```python
from build123d import *

# Parameters (mm, degrees)
F0_W           = 203.2
F0_H           = 88.9
F1_DEPTH       = 2.54
F2_W           = 2.54
F2_H           = 26.416
F2_H_2         = 2.54
F2_W_2         = 16.764
F2_W_3         = 26.416
F3_DEPTH       = 20.32
F5_D           = 3.048
F5_CSINK_D     = 5.08
F5_CSINK_ANGLE = 49
F2_W_4         = 85.8261585236
F2_H_3         = 19.05
F6_DEPTH       = 25.4
F7_SIZE2       = 19.5063104746
F7_SIZE        = 15.24


with BuildPart() as f1:
    # F0 (on Top) → F1 (new body)
    with BuildSketch(Plane.XY):
        Rectangle(F0_W, F0_H)
    extrude(amount=F1_DEPTH)

    # F2 (on face) → F3 (join)
    with BuildSketch(Plane.XY.offset(2.54)):
        with Locations((-33.782, -31.242)):
            Rectangle(F2_W, F2_H)
        with Locations((-53.086, -31.242)):
            Rectangle(F2_W, F2_H)
        with Locations((-53.086, -16.764)):
            Rectangle(F2_W, F2_H_2)
        with Locations((33.782, -31.242)):
            Rectangle(F2_W, F2_H)
        with Locations((53.086, -31.242)):
            Rectangle(F2_W, F2_H)
        with Locations((53.086, -16.764)):
            Rectangle(F2_W, F2_H_2)
        with Locations((-24.13, -16.764)):
            Rectangle(F2_W_2, F2_H_2)
        with Locations((-14.478, -16.764)):
            Rectangle(F2_W, F2_H_2)
        with Locations((24.13, -16.764)):
            Rectangle(F2_W_2, F2_H_2)
        with Locations((14.478, -16.764)):
            Rectangle(F2_W, F2_H_2)
        with Locations((-33.782, -16.764)):
            Rectangle(F2_W, F2_H_2)
        with Locations((-43.434, -16.764)):
            Rectangle(F2_W_2, F2_H_2)
        with Locations((33.782, -16.764)):
            Rectangle(F2_W, F2_H_2)
        with Locations((43.434, -16.764)):
            Rectangle(F2_W_2, F2_H_2)
        with Locations((0, -16.764)):
            Rectangle(F2_W_3, F2_H_2)
        Polygon((13.208, -37.338), (13.208, -44.45), (15.748, -44.45), (15.748, -18.034), (13.208, -18.034), (13.208, -34.798), align=None)
        Polygon((-15.748, -18.034), (-15.748, -44.45), (-13.208, -44.45), (-13.208, -37.338), (-13.208, -34.798), (-13.208, -18.034), align=None)
        with Locations((0, -36.068)):
            Rectangle(F2_W_3, F2_H_2)
    extrude(amount=F3_DEPTH)

    # F5 (through all)
    with Locations(Plane(origin=(0, 0, 0), x_dir=(1, 0, 0), z_dir=(0, 0, -1))):
        with Locations((97.155, -40.005), (97.155, 40.005), (-97.155, 40.005), (-97.155, -40.005)):
            CounterSinkHole(F5_D / 2, F5_CSINK_D / 2, counter_sink_angle=F5_CSINK_ANGLE)

    # F2 (on face) → F6 (join)
    with BuildSketch(Plane.XY.offset(2.54)):
        with Locations((0, 34.925)):
            Rectangle(F2_W_4, F2_H_3)
    extrude(amount=F6_DEPTH)

    # F7
    f7_edges = [f1.edges().sort_by_distance(p)[0] for p in [
        (0, 25.4, 27.94),
    ]]
    f7_side = f1.faces().sort_by_distance((0, 34.925, 27.94))[0]
    chamfer(f7_edges, length=F7_SIZE, length2=F7_SIZE2, reference=f7_side)


solid = f1.part
```
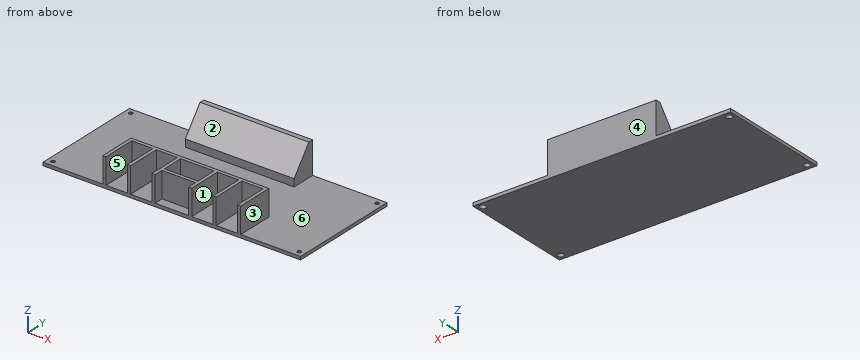
Design review of the part built by this model. Coordinates are the model's own, in mm. Face numbers are marked on the shaded views. A direction names the side the tool comes from. Round coordinates to 2 decimals unless told otherwise and drop trailing zeros. Write each loop counter-clockwise with the first axis right and the second up, starting at its lowest first coordinate (ties: lowest second). Pieces come first, ordered by that corner, then holes. Notation, with made-up numbers: (-35.5, -37.5) -> (-10.5, -37.5) arc R7 cw to (-10.5, -29.5) -> close; hole circle Ø4 at (-17, 40.5). An arc over 180 degrees is marked (long way). Write item = value, one per line. Start each with the question number.
1) Mouldability with a two-part tool opening along Y and no side actions: class the marked faces 4, 5 and 6 as +Y half, -Y half, draft (parallel to the pull), parting line (faces both ways), or undercut.
2) Take a section at C-C, the plane y = 29. State the section outline as (x, z) points, plus the area to 3 significant figures.
3) Clearance check with flat-ended pins moving along their axes: pin 1 (13.5 mm diameter, centred on x = -42, y = -31.5, fed in from +Z); pin 2 (2 mm diameter, centred on y = -22.5, z = 7, fed in from +X); pin 3 (6 mm diameter, centred on y = -32, z = 9, fed in from -X); pin 4 (13.5 mm diameter, centred on x = 26, z = 8.5, fed in from -Y). State where each tip first meets the part, or that it passes through.
4) Wall thickness on probe 1 along X at (y, z) = (-23, 7); probe 2 along X at (y, z) = (34, 9); probe 3 along Z at (x, y) = (75, -37): over which ranges is each line inside the solid? List them lowest first. Write a range as from..to.
5) Take a section at D-D, the plane y = -20. State the section outline as (x, z) points, plus the area to 3 significant figures.
6) Tool access review of the marked faces 1, 2 and 3: name each direction out of +Z, -Z, +X, -X, +Y, -Y from which nothing blocks a thin tool from reaching the whole face with its end or side.
7) Take a section at B-B, the plane x = 41. State the section outline as (y, z) points, plus the area to 3 significant figures.
8) Take a section at A-A, the plane z = 15.75. Count the separate pieces of the cut face and the enclosed holes in it, plus the area to 3 significant figures.
Results list:
q1.face_4 = +Y half
q1.face_5 = draft
q1.face_6 = undercut
q2.outline = (-101.6, 0) -> (101.6, 0) -> (101.6, 2.54) -> (42.91, 2.54) -> (42.91, 13.04) -> (-42.91, 13.04) -> (-42.91, 2.54) -> (-101.6, 2.54) -> close
q2.area = 1,420 mm²
q3.pin_1 = 2.54
q3.pin_2 = 54.36
q3.pin_3 = -54.36
q3.pin_4 = -44.45
q4.probe_1 = -54.36..-51.82, -35.05..-32.51, -15.75..-13.21, 13.21..15.75, 32.51..35.05, 51.82..54.36
q4.probe_2 = -42.91..42.91
q4.probe_3 = 0..2.54
q5.outline = (-101.6, 0) -> (101.6, 0) -> (101.6, 2.54) -> (54.36, 2.54) -> (54.36, 22.86) -> (51.82, 22.86) -> (51.82, 2.54) -> (35.05, 2.54) -> (35.05, 22.86) -> (32.51, 22.86) -> (32.51, 2.54) -> (15.75, 2.54) -> (15.75, 22.86) -> (13.21, 22.86) -> (13.21, 2.54) -> (-13.21, 2.54) -> (-13.21, 22.86) -> (-15.75, 22.86) -> (-15.75, 2.54) -> (-32.51, 2.54) -> (-32.51, 22.86) -> (-35.05, 22.86) -> (-35.05, 2.54) -> (-51.82, 2.54) -> (-51.82, 22.86) -> (-54.36, 22.86) -> (-54.36, 2.54) -> (-101.6, 2.54) -> close
q5.area = 826 mm²
q6.face_1 = +Z, -Y
q6.face_2 = +Z, +X, -X
q6.face_3 = +Z, +X, +Y, -Y
q7.outline = (-44.45, 0) -> (44.45, 0) -> (44.45, 27.94) -> (40.64, 27.94) -> (25.4, 8.43) -> (25.4, 2.54) -> (-15.49, 2.54) -> (-15.49, 22.86) -> (-18.03, 22.86) -> (-18.03, 2.54) -> (-44.45, 2.54) -> close
q7.area = 613 mm²
q8.separate_pieces = 2
q8.enclosed_holes = 1
q8.area = 1,890 mm²
